Check sheet for the modelled part. Datum: model origin and axes. Units: mm. Round coordinates to 2 decimals unless told otherwise and drop trailing zeros. Order: outer loops, then holes, each group sorted by start corner. A loop starts at its lowest first (then second) coordinate and runs counter-clockwise, first axis right, second up. Notation, with made-up numbers: (-34.5, -12) -> (11.5, -12) arc R16 cw to (11.5, 12) -> close; hole circle Ø4 at (83, -33.75). An arc over 180 degrees is marked (long way). Answer in a Markdown table with one row per item.
Autodesk Inventor part; units mm, degrees
ref_plane "YZ Plane" through (0, 0, 0) normal (1, 0, 0) x (0, 1, 0)
ref_plane "XZ Plane" through (0, 0, 0) normal (0, 1, 0) x (-1, 0, 0)
ref_plane "XY Plane" through (0, 0, 0) normal (0, 0, 1) x (1, 0, 0)
sketch "Boceto1" plane through (0, 0, 0) normal (0, 1, 0) x (-1, 0, 0)
  line L0 (0, 0) -> (0, -52.2241) construction
  line L1 (0, 0) -> (0, 54.663) construction
  line L2 (0, 0) -> (-57.9564, 0) construction
  line L3 (0, 0) -> (56.3387, 0) construction
  line L4 (-70, -20) -> (-40, -20)
  line L5 (-40, -20) -> (-40, 20)
  line L6 (-40, 20) -> (-70, 20)
  line L7 (-70, 20) -> (-70, -20)
  line L8 (-70, -20) -> (-40, 20) construction
  line L9 (-40, -20) -> (-70, 20) construction
  line L10 (-18, 63.0769) -> (-64.0145, 27.7688)
  line L11 (9, 69.9829) -> (55.0145, 34.6747)
  line L12 (9, 69.9829) -> (17.2117, 80.6846)
  line L13 (-18, 63.0769) -> (-28.8943, 77.2746)
  line L14 (-64.0145, 27.7688) -> (-72.6721, 39.0515)
  line L15 (-18, -63.0769) -> (-64.0145, -27.7688)
  line L16 (9, -69.9829) -> (55.0145, -34.6747)
  line L17 (9, -69.9829) -> (17.2117, -80.6846)
  line L18 (-18, -63.0769) -> (-28.8943, -77.2746)
  line L19 (-64.0145, -27.7688) -> (-72.6721, -39.0515)
  arc A0 (-72.6721, 39.0515) -> (-72.6721, -39.0515) centre (0, 0) ccw
  arc A1 (17.2117, 80.6846) -> (-28.8943, 77.2746) centre (0, 0) ccw
  arc A2 (-28.8943, -77.2746) -> (17.2117, -80.6846) centre (0, 0) ccw
  line L20 (59, 37.9189) -> (59, -37.9189)
  line L21 (58.0583, 38.6415) -> (59, 37.9189)
  line L22 (55.0145, 34.6747) -> (58.0583, 38.6415)
  line L23 (58.0583, -38.6415) -> (59, -37.9189)
  line L24 (55.0145, -34.6747) -> (58.0583, -38.6415)
  circle A3 centre (-18.868, 51.0667) radius 1.5
  circle A4 centre (-52.1888, 25.4987) radius 1.5
  line L25 (-41.0072, 45.4229) -> (-35.5284, 38.2827) construction
  line L26 (-18.868, 51.0667) -> (-52.1888, 25.4987) construction
  line L27 (32.0072, 52.3288) -> (22.9685, 40.5493) construction
  circle A5 centre (9.868, 57.9726) radius 1.5
  circle A6 centre (43.1888, 32.4046) radius 1.5
  circle A7 centre (-18.868, -51.0667) radius 1.5
  circle A8 centre (-52.1888, -25.4987) radius 1.5
  circle A9 centre (9.868, -57.9726) radius 1.5
  circle A10 centre (43.1888, -32.4046) radius 1.5
  line L28 (43.1888, 32.4046) -> (9.868, 57.9726) construction
  point P0 (-55, 0)
  point P1 (-70, 0)
  point P2 (26.5284, 45.1886)
  dimension "d1" = 30
  dimension "d2" = 40
  dimension "d3" = 70
  dimension "d9" = 52.5
  dimension "d10" = 52.5
  dimension "d11" = 61
  dimension "d12" = 61
  dimension "d13" = 58
  dimension "d17" = 90
  dimension "d18" = 9
  dimension "d19" = 18
  dimension "d20" = 58
  dimension "d21" = 90
  dimension "d22" = 90
  dimension "d23" = 82.5
  dimension "d24" = 82.5
  dimension "d26" = 59
  dimension "d27" = 5
  dimension "d28" = 5
  dimension "d29" = 3
  dimension "d30" = 3
  dimension "d31" = 42
  dimension "d32" = 9
  dimension "d37" = 90
  dimension "d38" = 3
  dimension "d39" = 3
  dimension "d40" = 42
  dimension "d41" = 9
extrude "Extrusión1" add sketch "Boceto1" along normal blind 3
sketch "Boceto2" plane through (0, 3, 0) normal (0, 1, 0) x (1, 0, 0)
  line L0 (-55.0145, -34.6747) -> (-9, -69.9829)
  line L1 (-32.0072, -52.3288) -> (-0.1642, -10.8301) construction
  circle A0 centre (-33.4486, -19.711) radius 1.55
  circle A1 centre (-0.1278, -45.2789) radius 1.55
  line L2 (-33.4486, -19.711) -> (-0.1278, -45.2789) construction
  circle A2 centre (-43.1888, -32.4046) radius 1.5 construction
  line L3 (18, -63.0769) -> (64.0145, -27.7688)
  line L4 (41.0072, -45.4229) -> (14.3892, -10.7335) construction
  circle A3 centre (9.1278, -38.373) radius 1.55
  circle A4 centre (42.4486, -12.805) radius 1.55
  line L5 (42.4486, -12.805) -> (9.1278, -38.373) construction
  circle A5 centre (18.868, -51.0667) radius 1.5 construction
  line L6 (-59, 37.9189) -> (-59, -37.9189) construction
  line L7 (-59, 0) -> (115.874, 0) construction
  circle A6 centre (-33.4486, 19.711) radius 1.55
  circle A7 centre (-0.1278, 45.2789) radius 1.55
  circle A8 centre (9.1278, 38.373) radius 1.55
  circle A9 centre (42.4486, 12.805) radius 1.55
  point P0 (0, 0)
  dimension "d44" = 3.1
  dimension "d45" = 3.1
  dimension "d46" = 21
  dimension "d47" = 42
  dimension "d48" = 16
  dimension "d51" = 16
  dimension "d52" = 21
  dimension "d53" = 42
extrude "Extrusión2" cut sketch "Boceto2" against normal blind 10
properties part number "newbasecentral"
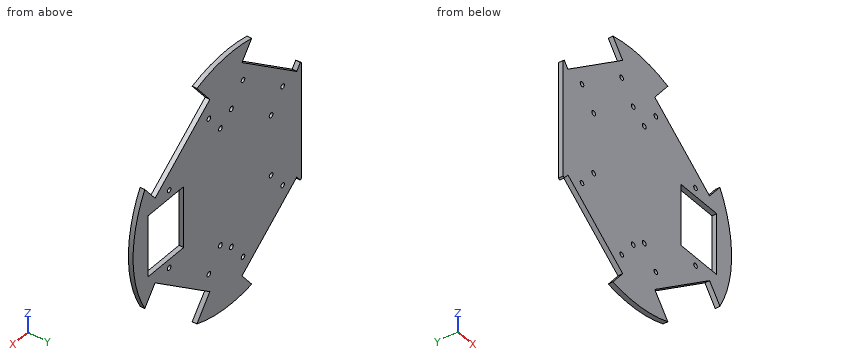
Item 1: Cross-section at A-A (x = 61.5). Record the boundary of the cut face in (y, z), and give its area (3 significant figures).
Result sheet:
| item | result |
|---|---|
| outline | (0, -29.7) -> (3, -29.7) -> (3, -20) -> (0, -20) -> close; (0, 20) -> (3, 20) -> (3, 29.7) -> (0, 29.7) -> close |
| area | 58.2 mm^2 |
Item 2: Depth check by flat-ended pin: P1, Ø12, axis at x = -43.5, z = -36, coming from the -Y side; P2, Ø0.9, axis at x = 55.5, y = 1, coming from the +Z side; P3, Ø2.5, axis at x = 52.19, z = 25.5, coming from the -Y side; P4, Ø1.5, axis at y = 2, z = -4.5, coming from the +X side. Enter the tip coordinate at first touch or a pass-through.
Result sheet:
| item | result |
|---|---|
| P1 | stops at y = 0 |
| P2 | stops at z = 34.65 |
| P3 | passes through |
| P4 | stops at x = 82.41 |
Item 3: Cross-section at C-C (x = 22.5). Record the boundary of the cut face in (y, z).
Result sheet:
| item | result |
|---|---|
| outline | (0, -79.37) -> (3, -79.37) -> (3, -68.94) -> (0, -68.94) -> close; (0, -59.62) -> (3, -59.62) -> (3, 59.62) -> (0, 59.62) -> close; (0, 68.94) -> (3, 68.94) -> (3, 79.37) -> (0, 79.37) -> close |
Item 4: Scan lines: line 1 (Z direction, x = 0, y = 2.8); line 2 (Z direction, x = -11, y = 1.2); line 3 (Z direction, x = -17, y = 2.65). Record each from-to range of solid material in increasing order. Write a range as [from, to].
Result sheet:
| item | result |
|---|---|
| line 1 | z = [-82.5, -46.82], [-43.73, 43.73], [46.82, 82.5] |
| line 2 | z = [-81.76, -72.59], [-68.45, -58.96], [-56.99, 56.99], [58.96, 68.45], [72.59, 81.76] |
| line 3 | z = [-80.73, -80.41], [-63.84, 63.84], [80.41, 80.73] |
Item 5: Cross-section at B-B (z = -10). Record the boundary of the cut face in (x, y), and give its area (3 significant figures).
Result sheet:
| item | result |
|---|---|
| outline | (-59, 0) -> (40, 0) -> (40, 3) -> (-59, 3) -> close; (70, 0) -> (81.89, 0) -> (81.89, 3) -> (70, 3) -> close |
| area | 333 mm^2 |
Item 6: Cross-section at D-D (y = 2.5). State how many separate pieces and enclosed holes the cut face has, and give its area (3 significant figures).
Result sheet:
| item | result |
|---|---|
| separate pieces | 1 |
| enclosed holes | 15 |
| area | 13,800 mm^2 |
